Read the model definition and answer for the solid it produces. Units are mm, in the model's axes. A direction names the side the tool comes from. Round coordinates to 2 decimals unless told otherwise and drop trailing zeros. Write each loop counter-clockwise with the first axis right and the second up, starting at its lowest first coordinate (ties: lowest second). Pieces come first, ordered by that corner, then holes.
from build123d import *

# Parameters (mm, degrees)
ESQUISSE1_W             = 50.3
ESQUISSE1_H             = 50.3
BOSS_EXTRU_1_DEPTH      = 6
BOSS_EXTRU_2_DEPTH      = 20
ESQUISSE3_R             = 1.5
ENL_V_MAT_EXTRU_1_DEPTH = 76.737573238
CONG_2_R                = 5
ESQUISSE4_R             = 4
ENL_V_MAT_EXTRU_2_DEPTH = 3
CONG_6_R                = 5
ESQUISSE5_R             = 16
ENL_V_MAT_EXTRU_3_DEPTH = 1
ESQUISSE6_R             = 15
ENL_V_MAT_EXTRU_4_DEPTH = 21


with BuildPart() as part:
    # Esquisse1 → Boss.-Extru.1 (new body)
    with BuildSketch(Plane.XY):
        with Locations((25.15, 25.15)):
            Rectangle(ESQUISSE1_W, ESQUISSE1_H)
    extrude(amount=BOSS_EXTRU_1_DEPTH)

    # Esquisse2 → Boss.-Extru.2 (add)
    with BuildSketch(Plane.XY.offset(6)):
        Polygon((4, 46.3), (46.3, 46.3), (46.3, 4), (33.3, 4), (33.3, 0), (50.3, 0), (50.3, 50.3), (0, 50.3), (0, 0), (17, 0), (17, 4), (4, 4), align=None)
    extrude(amount=BOSS_EXTRU_2_DEPTH)

    # Esquisse3 → Enlèv. mat.-Extru.1 (cut, through all)
    with BuildSketch(Plane(origin=(0, 0, 0), x_dir=(-1, 0, 0), z_dir=(0, 0, -1))):
        with Locations((-39.3, 39.6)):
            Circle(ESQUISSE3_R)
        with Locations((-14.3, 39.6)):
            Circle(ESQUISSE3_R)
        with Locations((-14.3, 9.6)):
            Circle(ESQUISSE3_R)
        with Locations((-39.3, 9.6)):
            Circle(ESQUISSE3_R)
    extrude(amount=-ENL_V_MAT_EXTRU_1_DEPTH, mode=Mode.SUBTRACT)

    # Congé2
    cong_2_edges = [part.edges().sort_by_distance(p)[0] for p in [
        (0, 50.3, 13),
    ]]
    fillet(cong_2_edges, radius=CONG_2_R)

    # Esquisse4 → Enlèv. mat.-Extru.2 (cut)
    with BuildSketch(Plane.XY.offset(6)):
        with Locations((14.3, 39.6)):
            Circle(ESQUISSE4_R)
        with Locations((39.3, 39.6)):
            Circle(ESQUISSE4_R)
        with Locations((39.3, 9.6)):
            Circle(ESQUISSE4_R)
        with Locations((14.3, 9.6)):
            Circle(ESQUISSE4_R)
    extrude(amount=-ENL_V_MAT_EXTRU_2_DEPTH, mode=Mode.SUBTRACT)

    # Congé6
    cong_6_edges = [part.edges().sort_by_distance(p)[0] for p in [
        (50.3, 50.3, 13),
        (50.3, 0, 13),
        (0, 0, 13),
    ]]
    fillet(cong_6_edges, radius=CONG_6_R)

    # Esquisse5 → Enlèv. mat.-Extru.3 (cut)
    with BuildSketch(Plane.XY.offset(6)):
        with Locations((26.8, 24.6)):
            Circle(ESQUISSE5_R)
    extrude(amount=-ENL_V_MAT_EXTRU_3_DEPTH, mode=Mode.SUBTRACT)

    # Esquisse6 → Enlèv. mat.-Extru.4 (cut)
    with BuildSketch(Plane.XY.offset(5)):
        with Locations((26.8, 24.6)):
            Circle(ESQUISSE6_R)
    extrude(amount=-ENL_V_MAT_EXTRU_4_DEPTH, mode=Mode.SUBTRACT)


solid = part.part
Q1. Straight lines are drawn through the part: probe 1 along Y at (x, z) = (37, 6.25); probe 2 along Y at (x, z) = (14.3, 5.05). For each, find the intervals that lie inside material, in ascending order.
Verdict:
probe 1: y = 0 to 4, 46.3 to 50.3
probe 2: y = 0 to 5.6, 13.6 to 14.61, 34.59 to 35.6, 43.6 to 50.3
Q2. Determine the mould class of faces 4 (the cylindrical face through (40.8, 9.67, 1.48)), 5 (the cylindrical face through (48.87, 1.5, 13.18)), 6 (the cylindrical face through (1, 2, 13)) for opening direction X: pulls with the +X half, pulls with the -X half, needs draft (parallel to the pull), parting line crosses it, or undercut.
Verdict:
face 4: undercut
face 5: pulls with the +X half
face 6: pulls with the -X half
Q3. Section C-C (x = 26) is taken. Determine the outline of the cut face in (y, z), then the cut area to 3 significant figures.
Verdict:
outline: (0, 0) - (9.62, 0) - (9.62, 5) - (8.62, 5) - (8.62, 6) - (0, 6) - close; (39.58, 0) - (50.3, 0) - (50.3, 26) - (46.3, 26) - (46.3, 6) - (40.58, 6) - (40.58, 5) - (39.58, 5) - close
area: 200 mm2
Q4. Which of the six approach directions +Z, -Z, +X, -X, +Y, -Y give full straight-line access (tool end or side, diameter ignored) to faces 1 (the cylindrical face through (43.115, 40.801, 4.521)), 2 (the cylindrical face through (40.41, 40.61, 1.48)), 3 (the flat face through (33.3, 2, 16))?
Verdict:
face 1: +Z
face 2: +Z, -Z
face 3: +Z, -Y
Q5. Flat-ended cylindrical pins translate along their axes: pin 1 Ø4 at (x, y) = (39.3, 9.6) entering from +Z; pin 2 Ø1.2 at (y, z) = (1.5, 15.5) entering from +X; pin 3 Ø10.5 at (x, y) = (39.3, 39.6) entering from +Z; pin 4 Ø1.5 at (x, y) = (22, 36.5) entering from -Z. Find the tip coordinate at first contact, or state that the pin passes through.
Verdict:
pin 1: stops at z = 3
pin 2: stops at x = 49.37
pin 3: stops at z = 6
pin 4: passes through
Q6. Section D-D (z = 12.75) is taken. Determine the outline of the cut face in (x, y).
Verdict:
outline: (0, 5) arc R5 ccw to (5, 0) - (17, 0) - (17, 4) - (4, 4) - (4, 46.3) - (46.3, 46.3) - (46.3, 4) - (33.3, 4) - (33.3, 0) - (45.3, 0) arc R5 ccw to (50.3, 5) - (50.3, 45.3) arc R5 ccw to (45.3, 50.3) - (5, 50.3) arc R5 ccw to (0, 45.3) - close
Q7. Section A-A (y = 24.6) is taken. Determine the outline of the cut face in (x, z).
Verdict:
outline: (0, 0) - (11.8, 0) - (11.8, 5) - (10.8, 5) - (10.8, 6) - (4, 6) - (4, 26) - (0, 26) - close; (41.8, 0) - (50.3, 0) - (50.3, 26) - (46.3, 26) - (46.3, 6) - (42.8, 6) - (42.8, 5) - (41.8, 5) - close
Q8. Section B-B (x = 7) is taken. Determine the outline of the cut face in (y, z).
Verdict:
outline: (0, 0) - (50.3, 0) - (50.3, 26) - (46.3, 26) - (46.3, 6) - (4, 6) - (4, 26) - (0, 26) - close
